Can you work these out from the model? Positions are in its coordinate system, mm. Coordinates: 2 decimals unless noted, no trailing zeros. Loops run counter-clockwise (first coordinate to the right, second up) from the corner with the lowest first, then second, coordinate; pieces in that order, holes last.
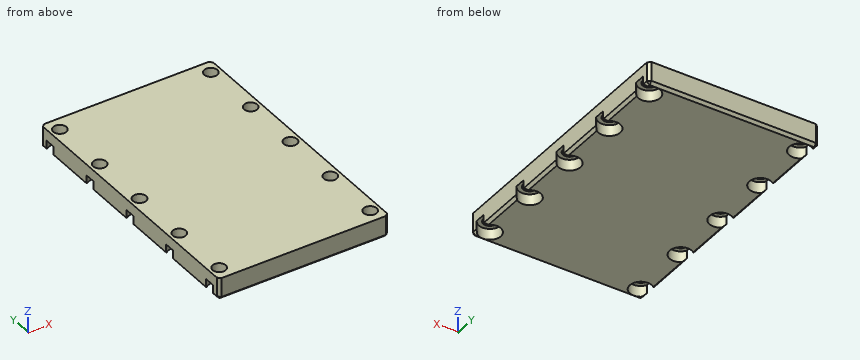
```python
from build123d import *

# Parameters (mm, degrees)
SKETCH_1_W                   = 62
SKETCH_1_H                   = 98
EXTRUDE_1_DEPTH              = 8
CHAMFER_1_SIZE               = 1
HOLE_WIZARD_M4_1_D           = 4.8
HOLE_WIZARD_M4_1_CBORE_D     = 8
HOLE_WIZARD_M4_1_CBORE_DEPTH = 4
MIRROR_2_COPY_1_D            = 4.8
MIRROR_2_COPY_1_CBORE_D      = 8
MIRROR_2_COPY_1_CBORE_DEPTH  = 4


with BuildPart() as part:
    # ｽｹｯﾁ1 → ﾎﾞｽ - 押し出し1 (new body)
    with BuildSketch(Plane.XY):
        Rectangle(SKETCH_1_W, SKETCH_1_H)
    extrude(amount=EXTRUDE_1_DEPTH)

    # 面取り1
    chamfer_1_edges = [part.edges().sort_by_distance(p)[0] for p in [
        (0, -49, 0),
        (-31, 0, 0),
        (0, 49, 0),
        (31, 0, 0),
        (31, -49, 4),
        (-31, -49, 4),
        (-31, 49, 4),
        (31, 49, 4),
    ]]
    chamfer(chamfer_1_edges, length=CHAMFER_1_SIZE)

    # M4 穴付きねじ用座ぐり穴1 (through all)
    with Locations(Plane(origin=(0, 0, 0), x_dir=(1, 0, 0), z_dir=(0, 0, -1))):
        with Locations((-27.5, -44), (-27.5, -22), (-27.5, 0)):
            hole_wizard_m4_1 = CounterBoreHole(HOLE_WIZARD_M4_1_D / 2, HOLE_WIZARD_M4_1_CBORE_D / 2, HOLE_WIZARD_M4_1_CBORE_DEPTH)

    # ﾐﾗｰ1: M4 穴付きねじ用座ぐり穴1 across plane
    add(hole_wizard_m4_1.mirror(Plane.ZX), mode=Mode.SUBTRACT)

    # ﾐﾗｰ2: M4 穴付きねじ用座ぐり穴1 across plane
    add(hole_wizard_m4_1.mirror(Plane(origin=(0, 0, 0), x_dir=(0, 0, 1), z_dir=(1, 0, 0))), mode=Mode.SUBTRACT)

    # ﾐﾗｰ2 copy 1 (through all)
    with Locations(Plane(origin=(0, 0, 0), x_dir=(-1, 0, 0), z_dir=(0, 0, -1))):
        with Locations((-27.5, -44), (-27.5, -22), (-27.5, 0)):
            CounterBoreHole(MIRROR_2_COPY_1_D / 2, MIRROR_2_COPY_1_CBORE_D / 2, MIRROR_2_COPY_1_CBORE_DEPTH)


solid = part.part
```
(1) I want a section at A-A on y = 22. Write out the boundary of the cut face in (x, z).
Check values:
outline: (-31, 4) - (-29.9, 4) - (-29.9, 8) - (-31, 8) - close; (-25.1, 4) - (-23.5, 4) - (-23.5, 0) - (23.5, 0) - (23.5, 4) - (25.1, 4) - (25.1, 8) - (-25.1, 8) - close; (29.9, 4) - (31, 4) - (31, 8) - (29.9, 8) - close
(2) I'm going to push flat-ended pins straight in: pin 1 (4 mm diameter, centred on x = 27.5, y = 22, fed in from +Z); pin 2 (4 mm diameter, centred on x = 27, y = 44.5, fed in from -Z). Where does each tip first touch, or does it pass through?
Check values:
pin 1: passes through
pin 2: stops at z = 4
(3) If I drill on probe 1 along X at (y, z) = (44, 4.95); probe 2 along Y at (x, z) = (-27.5, 2.75); probe 3 along Y at (x, z) = (24, 2), over which ranges is the centre line in solid material (lowest first)?
Check values:
probe 1: x = -31 to -29.9, -25.1 to 25.1, 29.9 to 31
probe 2: y = -49 to -48, -40 to -26, -18 to -4, 4 to 18, 26 to 40, 48 to 49
probe 3: y = -49 to -45.94, -42.06 to -23.94, -20.06 to -1.94, 1.94 to 20.06, 23.94 to 42.06, 45.94 to 49
(4) I want a section at B-B on z = 6.75. State how many separate pieces and enclosed holes the cut face has, then the cut area to 3 significant figures.
Check values:
separate pieces: 1
enclosed holes: 10
area: 5,890 mm2
